The model under review builds one solid part; all positions refer to its coordinate system, in mm. A direction names the side the tool comes from. Give positions to 0.01 mm unless a question says otherwise; leave off trailing zeros. Loops run counter-clockwise (first coordinate to the right, second up) from the corner with the lowest first, then second, coordinate; pieces in that order, holes last. Notation, with made-up numbers: M 50.5,79 L 96.5,79 A27 cw 96.5,114 Z; hole C 3.25,50 d7. An arc over 180 degrees is marked long. Put each result on its own line as item: value. Start each with the question number.
Autodesk Inventor part; units mm, degrees
ref_plane "YZ Plane" through (0, 0, 0) normal (1, 0, 0) x (0, 1, 0)
ref_plane "XZ Plane" through (0, 0, 0) normal (0, 1, 0) x (-1, 0, 0)
ref_plane "XY Plane" through (0, 0, 0) normal (0, 0, 1) x (1, 0, 0)
sketch "Sketch1" plane through (0, 0, 0) normal (0, 0, 1) x (1, 0, 0)
  line L0 (0, 0) -> (50.8, 0)
  line L1 (50.8, 0) -> (50.8, 101.6)
  line L2 (50.8, 101.6) -> (0, 101.6)
  line L3 (0, 101.6) -> (0, 0)
  dimension "d0" = 101.6
  dimension "d1" = 50.8
extrude "Extrusion1" add sketch "Sketch1" along normal blind 1371.6
shell "Shell1" thickness 3.175 removed faces 2 at (16.9333, 67.7333, 0) at (16.9333, 67.7333, 1371.6)
fillet "Fillet1" radius 6.35 8 edges at (3.175, 3.175, 685.8) (47.625, 3.175, 685.8) (3.175, 98.425, 685.8) (47.625, 98.425, 685.8) (50.8, 101.6, 685.8) (50.8, 0, 685.8) (0, 0, 685.8) (0, 101.6, 685.8)
sketch "Sketch2" plane through (6.35, 0, 0) normal (0, -1, 0) x (1, 0, 0)
  circle A0 centre (19.05, 63.1) radius 4
  circle A1 centre (19.05, 13.1) radius 4
  line L0 (19.05, 63.1) -> (19.05, 13.1) construction
  line L1 (0, 0) -> (38.1, 0) construction
  line L2 (38.1, 1371.6) -> (38.1, 0) construction
  line L3 (38.1, 685.8) -> (-101.1432, 685.8) construction
  circle A2 centre (19.05, 1308.5) radius 4
  circle A3 centre (19.05, 1358.5) radius 4
  point P0 (-6.35, 0)
  point P1 (19.05, 38.1)
  point P2 (19.05, 0)
  dimension "d6" = 8
  dimension "d7" = 38.1
  dimension "d8" = 50
extrude "Extrusion2" cut sketch "Sketch2" against normal blind 1244.6
properties part number "2x4_Tube"
Item 1: Consider section A-A, the plane y = 67. Write out the cut boundary in (x, z) (3 decimals), plus the area to 3 significant figures.
Item 2: Consider section B-B, the plane z = 142.5. Write out the cut boundary in (x, y) (3 decimals).
Item 3: Draft analysis for pull direction Y (two halves, no side actions). For faces 1 (the flat face through (25, 3.175, 676)), 2 (the flat face through (26, 101.6, 676)), 3 (the flat face through (0, 51, 676)), state which applies: +Y half, -Y half, draft (parallel to the pull), parting line (faces both ways), or undercut.
Item 4: Tool access review of faces 4 (the flat face through (3.175, 51, 676)), 5 (the flat face through (3, 51, 1371.6)): name each direction out of +Z, -Z, +X, -X, +Y, -Y from which nothing blocks a thin tool from reaching the whole face with its end or side.
Item 5: To check wall thickness, follow L1, parallel to Z at x = 25, y = 100; L2, parallel to X at y = 1, z = 1358; L3, parallel to X at y = 59, z = 806 (3 decimals). State the ranges of each line that lie inside material, in increasing order. Write a range as [from, to].
Report:
1. outline: M 0,0 L 3.175,0 L 3.175,1371.6 L 0,1371.6 Z; M 47.625,0 L 50.8,0 L 50.8,1371.6 L 47.625,1371.6 Z
1. area: 8,710 mm²
2. outline: M 0,6.35 A6.35 ccw 6.35,0 L 44.45,0 A6.35 ccw 50.8,6.35 L 50.8,95.25 A6.35 ccw 44.45,101.6 L 6.35,101.6 A6.35 ccw 0,95.25 Z; hole M 3.175,9.525 A6.35 ccw 9.525,3.175 L 41.275,3.175 A6.35 ccw 47.625,9.525 L 47.625,92.075 A6.35 ccw 41.275,98.425 L 9.525,98.425 A6.35 ccw 3.175,92.075 Z
3. face 1: undercut
3. face 2: +Y half
3. face 3: draft
4. face 4: +Z, -Z
4. face 5: +Z, +X, -X, +Y, -Y
5. L1: [0, 9.12], [17.08, 59.12], [67.08, 1304.52], [1312.48, 1354.52], [1362.48, 1371.6]
5. L2: [2.93, 21.43], [29.37, 47.87]
5. L3: [0, 3.175], [47.625, 50.8]
